Source: CAD feature listing. Evaluate the final solid. Frame: model axes, mm. Face numbers are marked on the shaded views. Give positions to 0.01 mm unless a question says otherwise; leave off trailing zeros. Order: outer loops, then holes, each group sorted by start corner. A loop starts at its lowest first (then second) coordinate and runs counter-clockwise, first axis right, second up.
from build123d import *

# Parameters (mm, degrees)
BOSS_EXTRU_1_DEPTH      = 4
ENL_V_MAT_EXTRU_1_REACH = 6
ESQUISSE2_R             = 2


with BuildPart() as part:
    # Esquisse1 → Boss.-Extru.1 (new body)
    with BuildSketch(Plane.XY):
        Polygon((0, 4.041451884), (-3.5, 2.020725942), (-3.5, -2.020725942), (0, -4.041451884), (3.5, -2.020725942), (3.5, 2.020725942), align=None)
    extrude(amount=BOSS_EXTRU_1_DEPTH)

    # Esquisse2 → Enlèv. mat.-Extru.1 (cut, up to next)
    with BuildSketch(Plane.XY.offset(4), mode=Mode.PRIVATE) as enl_v_mat_extru_1_sk1:
        Circle(ESQUISSE2_R)
    enl_v_mat_extru_1_tool1 = extrude(enl_v_mat_extru_1_sk1.sketch, amount=-ENL_V_MAT_EXTRU_1_REACH, mode=Mode.PRIVATE) & part.part
    add(enl_v_mat_extru_1_tool1.solids().sort_by_distance((0, 0, 4))[0], mode=Mode.SUBTRACT)

    # Esquisse4 → Enlèvement de matière-Révolution8 (revolve, cut)
    with BuildSketch(Plane(origin=(0, 0, 0), x_dir=(1, 0, 0), z_dir=(0, 1, 0))):
        Polygon((-6.964101615, -2), (-1.767949192, 1), (-7.964101615, 1), (-7.964101615, -5), (-1.767949192, -5), align=None)
    revolve(axis=Axis((0, 0, 0), (0, 0, 1)), mode=Mode.SUBTRACT)


solid = part.part
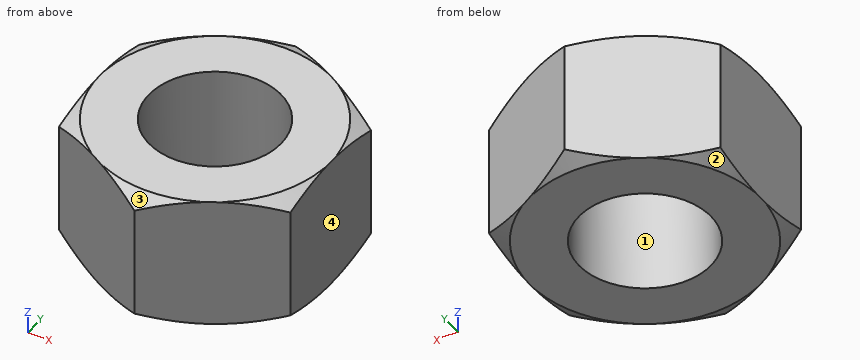
1) Section query A-A on z = 3.2. Output: boundary loops of the cut face in (x, y).
Checks:
outline: (-3.5, -2.02) - (0, -4.04) - (3.5, -2.02) - (3.5, 2.02) - (0, 4.04) - (-3.5, 2.02) - close; hole circle Ø4 at (0, 0)
2) Ray query, L1, parallel to X at y = -1.5, z = 1.85; L2, parallel to Y at x = -0.75, z = 1.8; L3, parallel to Y at x = -1.5, z = 2.95. Return the intervals inside material, ascending.
Checks:
L1: x = -3.5 to -1.32, 1.32 to 3.5
L2: y = -3.61 to -1.85, 1.85 to 3.61
L3: y = -3.18 to -1.32, 1.32 to 3.18
3) Pull-direction query (Y, two-part tool) for the marked faces 1, 2, 3 and 4; classes: +Y half, -Y half, draft (parallel to the pull), parting line (faces both ways), or undercut.
Checks:
face 1: undercut
face 2: +Y half
face 3: -Y half
face 4: draft
